from build123d import *

# Parameters (mm, degrees)
SKETCH1_W           = 13.97
SKETCH1_H           = 13.97
BOSS_EXTRUDE1_DEPTH = 6.35
SKETCH4_W           = 7.62
SKETCH4_H           = 33.02
SKETCH4_H_2         = 27.94
CUT_EXTRUDE1_DEPTH  = 176.747076789
SKETCH5_R           = 2.38125
CUT_EXTRUDE2_DEPTH  = 176.747076789


with BuildPart() as part:
    # Sketch1 → Boss-Extrude1 (new body)
    with BuildSketch(Plane(origin=(0, 0, 0), x_dir=(1, 0, 0), z_dir=(0, 1, 0))):
        with BuildLine():
            Line((-95.25, -38.1), (95.25, -38.1))
            ThreePointArc((95.25, -38.1), (133.35, 0), (95.25, 38.1))
            Line((95.25, 38.1), (57.15, 38.1))
            ThreePointArc((57.15, 38.1), (39.189487758, 45.539487758), (31.75, 63.5))
            Line((31.75, 63.5), (31.75, 88.9))
            ThreePointArc((31.75, 88.9), (24.310512242, 106.860512242), (6.35, 114.3))
            Line((6.35, 114.3), (-107.95, 114.3))
            ThreePointArc((-107.95, 114.3), (-125.910512242, 106.860512242), (-133.35, 88.9))
            Line((-133.35, 88.9), (-133.35, 0))
            ThreePointArc((-133.35, 0), (-122.190768363, -26.940768363), (-95.25, -38.1))
        make_face()
        Rectangle(SKETCH1_W, SKETCH1_H, mode=Mode.SUBTRACT)
        with BuildLine():
            Line((95.25, -3.96875), (69.85, -3.96875))
            ThreePointArc((69.85, -3.96875), (65.88125, 0), (69.85, 3.96875))
            Line((69.85, 3.96875), (95.25, 3.96875))
            ThreePointArc((95.25, 3.96875), (99.21875, 0), (95.25, -3.96875))
        make_face(mode=Mode.SUBTRACT)
        with BuildLine():
            Line((-95.25, -3.96875), (-69.85, -3.96875))
            ThreePointArc((-69.85, -3.96875), (-65.88125, 0), (-69.85, 3.96875))
            Line((-69.85, 3.96875), (-95.25, 3.96875))
            ThreePointArc((-95.25, 3.96875), (-99.21875, 0), (-95.25, -3.96875))
        make_face(mode=Mode.SUBTRACT)
    extrude(amount=BOSS_EXTRUDE1_DEPTH)

    # Sketch4 → Cut-Extrude1 (cut, through all)
    with BuildSketch(Plane(origin=(0, 6.35, 0), x_dir=(1, 0, 0), z_dir=(0, 1, 0))):
        with Locations((16.51, -8.382)):
            Rectangle(SKETCH4_W, SKETCH4_H)
        with Locations((-48.641, -8.382)):
            Rectangle(SKETCH4_W, SKETCH4_H)
        with Locations((16.51, 89.408)):
            Rectangle(SKETCH4_W, SKETCH4_H_2)
        with Locations((-48.641, 89.154)):
            Rectangle(SKETCH4_W, SKETCH4_H_2)
    extrude(amount=-CUT_EXTRUDE1_DEPTH, mode=Mode.SUBTRACT)

    # Sketch5 → Cut-Extrude2 (cut, through all)
    with BuildSketch(Plane(origin=(0, 6.35, 0), x_dir=(1, 0, 0), z_dir=(0, 1, 0))):
        with Locations(Location((-62.9158, 88.9, 0), (0, 0, 270))):
            Circle(SKETCH5_R)
        with Locations(Location((-62.9158, 18.455847939, 0), (0, 0, 270))):
            Circle(SKETCH5_R)
    extrude(amount=-CUT_EXTRUDE2_DEPTH, mode=Mode.SUBTRACT)


solid = part.part
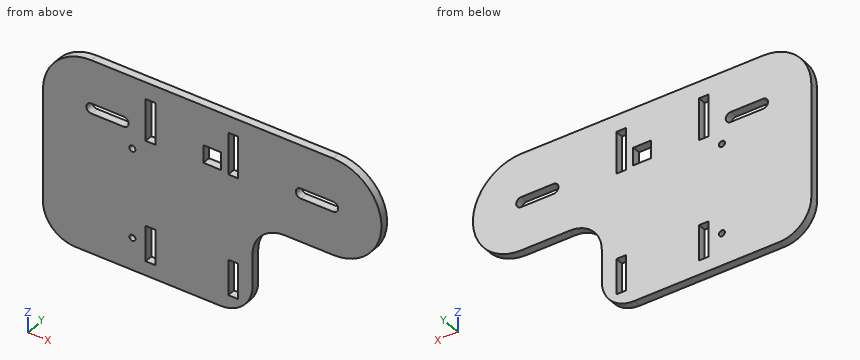
Read the model definition and answer for the solid it produces. Units are mm, in the model's axes. Round coordinates to 2 decimals unless told otherwise and drop trailing zeros. Order: outer loops, then holes, each group sorted by start corner. A loop starts at its lowest first (then second) coordinate and runs counter-clockwise, first axis right, second up.
1) Straight lines are drawn through the part: L1, parallel to X at y = 2, z = -88.9; L2, parallel to X at y = 0.5, z = -80; L3, parallel to X at y = 5, z = 10.5. For each, find the intervals that lie inside material, in ascending order.
2) The part is cut by section D-D on x = -111.5. Write down the section's boundary in (y, z), plus the area to 3 significant figures.
3) The part is cut by section C-C on y = 2.25. Give the number of separate pieces and of enclosed holes in the cut face, plus the area to 3 significant figures.
4) The part is cut by section B-B on z = -31. Write down the section's boundary in (x, y), plus the area to 3 significant figures.
5) Flat-ended cylindrical pins translate along their axes: pin 1 (3 mm diameter, centred on y = 3.5, z = 22.5, fed in from +X); pin 2 (1 mm diameter, centred on y = 3, z = -25.5, fed in from +X); pin 3 (1.9 mm diameter, centred on y = 4.5, z = 4, fed in from +X). Find the tip coordinate at first contact, or state that the pin passes through.
6) The part is cut by section A-A on x = 79. Write down the section's boundary in (y, z).
Resolved:
1. L1: x = -133.35 to -65.3, -60.53 to -52.45, -44.83 to 12.7, 20.32 to 31.75
1. L2: x = -133.35 to -52.45, -44.83 to 12.7, 20.32 to 31.75
1. L3: x = -131.87 to -52.45, -44.83 to 12.7, 20.32 to 131.87
2. outline: (0, -114.05) - (6.35, -114.05) - (6.35, 34.46) - (0, 34.46) - close
2. area: 943 mm2
3. separate pieces: 1
3. enclosed holes: 9
3. area: 30,200 mm2
4. outline: (-133.35, 0) - (117.4, 0) - (117.4, 6.35) - (-133.35, 6.35) - close
4. area: 1,590 mm2
5. pin 1: stops at x = 127.04
5. pin 2: stops at x = 124
5. pin 3: stops at x = 133.23
6. outline: (0, -38.1) - (6.35, -38.1) - (6.35, -3.97) - (0, -3.97) - close; (0, 3.97) - (6.35, 3.97) - (6.35, 38.1) - (0, 38.1) - close
